Can you work these out from the model? Positions are in its coordinate system, mm. Face numbers are marked on the shaded views. A direction names the side the tool comes from. Coordinates: 2 decimals unless noted, no trailing zeros. Write each loop counter-clockwise with the first axis right and the second up, starting at its lowest first coordinate (ties: lowest second). Pieces come first, ordered by that corner, then holes. Notation, with made-up numbers: (-31, 85) - (-1, 85) arc R16 ccw to (-1, 96) - close; hole circle Ø3 at (32, 59.25). An arc over 180 degrees is marked (long way). Use one line per item in the form item = value. Start each with the question number.
(1) If we section it at A-A on y = 25.5: Please give me the cut outline in (x, z), then the cut area to 3 significant figures.
(2) If we section it at B-B on z = -1: Please give me the cut outline in (x, y).
(3) On a 3-axis mill with a long thin cutter (end or side, diameter ignored), from which of +Z, -Z, +X, -X, +Y, -Y can I reach the whole of each face in a straight line? I mean the marked faces 5, 6, 7, 8 and 9. Say none if no direction works.
(4) Thinking about a two-plate mould opening in Z: for the marked faces 1, 2, 3 and 4, which applies, pulls with the +Z half, pulls with the -Z half, needs draft (parallel to the pull), parting line crosses it, or undercut?
(5) If I drill on probe 1 along X at (y, z) = (23, 0); probe 2 along X at (y, z) = (6.5, 1.5); probe 3 along Z at (x, y) = (15, 8), over which ranges is the centre line in solid material (lowest first)? Write a range as from..to.
(6) If we section it at D-D on y = 34.5: Please give me the cut outline in (x, z), then the cut area to 3 significant figures.
(7) If we section it at C-C on x = 0: Please give me the cut outline in (y, z), then the cut area to 3 significant figures.
Autodesk Inventor part; units mm, degrees
ref_plane "YZ Plane" through (0, 0, 0) normal (1, 0, 0) x (0, 1, 0)
ref_plane "XZ Plane" through (0, 0, 0) normal (0, 1, 0) x (-1, 0, 0)
ref_plane "XY Plane" through (0, 0, 0) normal (0, 0, 1) x (1, 0, 0)
sketch "Sketch1" plane through (0, 0, 0) normal (0, 1, 0) x (-1, 0, 0)
  line L0 (18, 18) -> (-18, 18)
  line L1 (-18, 18) -> (-18, -18)
  line L2 (-18, -18) -> (18, -18)
  line L3 (18, -18) -> (18, 18)
  line L4 (18, 18) -> (-18, -18) construction
  line L5 (-18, 18) -> (18, -18) construction
  point P0 (0, 0)
  dimension "d0" = 36
  dimension "d1" = 36
extrude "Extrusion1" add sketch "Sketch1" along normal blind 5
sketch "Sketch2" plane through (0, 5, 0) normal (0, 1, 0) x (1, 0, 0)
  line L0 (18, -18) -> (18, 18)
  line L1 (18, 18) -> (-18, 18)
  line L2 (-18, 18) -> (-18, -18)
  line L3 (-18, -18) -> (18, -18)
  line L4 (-18, -18) -> (18, -18)
  line L5 (18, -18) -> (18, 18)
  line L6 (18, 18) -> (-18, 18)
  line L7 (-18, 18) -> (-18, -18)
  line L8 (-18, -18) -> (18, 18) construction
  line L9 (18, -18) -> (-18, 18) construction
  point P0 (0, 0)
extrude "Extrusion2" add sketch "Sketch2" along normal blind 47
sketch "Sketch3" plane through (0, 52, 0) normal (0, 1, 0) x (1, 0, 0)
  line L0 (-15, 0) -> (15, 0) construction
  point P0 (0, 0)
  point P1 (0, 0)
  dimension "d6" = 30
hole "Hole1" at (-15, 52, 0) at (15, 52, 0) direction (0, -1, 0) diameter 5.2 end through all counterbore diameter 10 counterbore depth 19
fillet "Fillet1" radius 4 8 edges at (18, 26, 18) (-18, 26, 18) (18, 26, -18) (-18, 26, -18) (18, 42.5, -4) (18, 42.5, 4) (-18, 42.5, 4) (-18, 42.5, -4)
sketch "Sketch4" plane through (0, 52, 0) normal (0, 1, 0) x (1, 0, 0)
  point P0 (0, 0)
  point P1 (0, 0)
hole "Hole2" at (0, 52, 0) direction (0, -1, 0) diameter 5.2 depth 20
properties part number "LED Power Box (12V) Pillar" material "ABS Plastic"
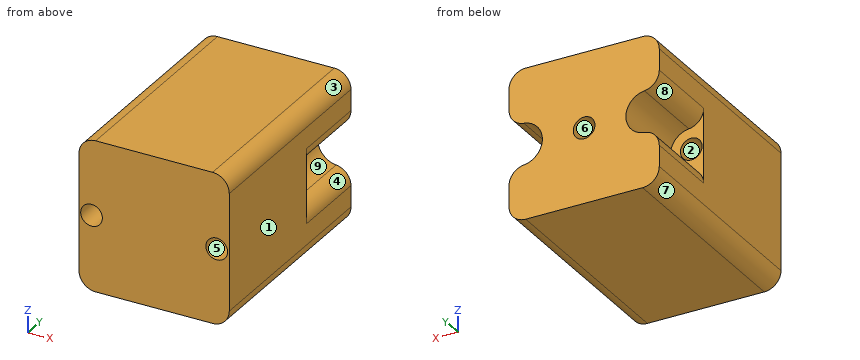
Reported:
q1.outline = (-18, -14) arc R4 ccw to (-14, -18) - (14, -18) arc R4 ccw to (18, -14) - (18, 14) arc R4 ccw to (14, 18) - (-14, 18) arc R4 ccw to (-18, 14) - close; hole circle Ø5.2 at (-15, 0); hole circle Ø5.2 at (15, 0)
q1.area = 1,240 mm2
q2.outline = (-18, 0) - (-17.4, 0) - (-17.4, 33) - (-18, 33) - close; (-12.6, 0) - (12.6, 0) - (12.6, 33) - (10.1, 33) - (10.1, 52) - (2.4, 52) - (2.4, 32) - (-2.4, 32) - (-2.4, 52) - (-10.1, 52) - (-10.1, 33) - (-12.6, 33) - close; (17.4, 0) - (18, 0) - (18, 33) - (17.4, 33) - close
q3.face_5 = +Y, -Y
q3.face_6 = +Y
q3.face_7 = -Z, -X, +Y, -Y
q3.face_8 = -X, +Y
q3.face_9 = +X, +Y
q4.face_1 = needs draft
q4.face_2 = undercut
q4.face_3 = pulls with the +Z half
q4.face_4 = undercut
q5.probe_1 = -18..-17.6, -12.4..12.4, 17.6..18
q5.probe_2 = -18..-17.12, -12.88..12.88, 17.12..18
q5.probe_3 = -17.87..-2.6, 2.6..17.87
q6.outline = (-18, -14) arc R4 ccw to (-14, -18) - (14, -18) arc R4 ccw to (18, -14) - (18, -8.94) arc R4 ccw to (14.44, -4.97) arc R5 cw to (14.44, 4.97) arc R4 ccw to (18, 8.94) - (18, 14) arc R4 ccw to (14, 18) - (-14, 18) arc R4 ccw to (-18, 14) - (-18, 8.94) arc R4 ccw to (-14.44, 4.97) arc R5 cw to (-14.44, -4.97) arc R4 ccw to (-18, -8.94) - close; hole circle Ø5.2 at (0, 0)
q6.area = 1,110 mm2
q7.outline = (0, -18) - (52, -18) - (52, -2.6) - (32, -2.6) - (32, 2.6) - (52, 2.6) - (52, 18) - (0, 18) - close
q7.area = 1,770 mm2
